```python
from build123d import *

# Parameters (mm, degrees)
CROQUIS3_W              = 31.215869756
CROQUIS3_H              = 35
SALIENTE_EXTRUIR3_DEPTH = 1.5


with BuildPart() as part:
    # Croquis3 → Saliente-Extruir3 (new, symmetric)
    with BuildSketch(Plane.XY):
        with Locations((-2.607934878, 2)):
            Rectangle(CROQUIS3_W, CROQUIS3_H)
        Polygon((-13.4988893, -15.5), (-13.58549184, -15.65), (-14.480384758, -17.2), (-8.210214166, -17.2), (-9.105107083, -15.65), (-9.191709623, -15.5), align=None)
        Polygon((6.117691454, -15.5), (1.810511777, -15.5), (1.723909236, -15.65), (0.829016319, -17.2), (7.099186911, -17.2), (6.204293994, -15.65), align=None)
        Polygon((13.15, 16.08549184), (13, 15.9988893), (13, 11.691709623), (13.15, 11.605107083), (14.7, 10.710214166), (14.7, 16.980384758), align=None)
        Polygon((13, -1.310511777), (13, -5.617691454), (13.15, -5.704293994), (14.7, -6.599186911), (14.7, -0.329016319), (13.15, -1.223909236), align=None)
    extrude(amount=SALIENTE_EXTRUIR3_DEPTH, both=True)


solid = part.part
```
Input: part model. Units: mm. Frame: model coordinates. A direction names the side the tool comes from. Give positions to 0.01 mm unless a question says otherwise; leave off trailing zeros. Loops run counter-clockwise (first coordinate to the right, second up) from the corner with the lowest first, then second, coordinate; pieces in that order, holes last.
1) Contact query for flat-ended pins moving along their axis: pin 1 (1.5 mm diameter, centred on y = 8, z = 0.5, fed in from +X); pin 2 (0.9 mm diameter, centred on x = 10.5, z = 0.5, fed in from -Y). Output: stop coordinate, or through.
A:
pin 1: stops at x = 13
pin 2: stops at y = -15.5
2) Mould query, pull axis X, two halves, no side actions, for faces 4 (the flat face through (-3, 19.5, 0)), 5 (the flat face through (14.7, 14, 0)), 6 (the flat face through (13, 18, 0)). Classes: released by +X, released by -X, zero draft, split by the parting line, or undercut.
A:
face 4: zero draft
face 5: released by +X
face 6: undercut
3) Section query C-C on x = -7.5. Return the cut outline in (y, z).
A:
outline: (-15.5, -1.5) - (19.5, -1.5) - (19.5, 1.5) - (-15.5, 1.5) - close
4) Reachability of faces 1 (the flat face through (-4, -15.5, 0)), 2 (the flat face through (-16, -15.5, 0)), 3 (the flat face through (-11, -17.2, 0)) from +Z, -Z, +X, -X, +Y, -Y: full face, straight path, thin tool, end or side. Return the list, or none.
A:
face 1: +Z, -Z
face 2: +Z, -Z, -X
face 3: +Z, -Z, +X, -X, -Y
5) Section query A-A on z = -1. Return the cut outline in (x, y).
A:
outline: (-18.22, -15.5) - (-13.5, -15.5) - (-14.48, -17.2) - (-8.21, -17.2) - (-9.19, -15.5) - (1.81, -15.5) - (0.83, -17.2) - (7.1, -17.2) - (6.12, -15.5) - (13, -15.5) - (13, -5.62) - (14.7, -6.6) - (14.7, -0.33) - (13, -1.31) - (13, 11.69) - (14.7, 10.71) - (14.7, 16.98) - (13, 16) - (13, 19.5) - (-18.22, 19.5) - close
6) Line query: L1, parallel to Y at x = -3, z = 0.95; L2, parallel to X at y = 18, z = -0.9; L3, parallel to Y at x = -8.5, z = -0.55. Output: solid intervals per line, ascending.
A:
L1: y = -15.5 to 19.5
L2: x = -18.22 to 13
L3: y = -17.2 to -16.7, -15.5 to 19.5
7) Section query B-B on y = -10. Return the cut outline in (x, z).
A:
outline: (-18.22, -1.5) - (13, -1.5) - (13, 1.5) - (-18.22, 1.5) - close
